```python
from build123d import *

# Parameters (mm, degrees)
RESSALTO_EXTRUS_O1_DEPTH   = 160
ESBO_O2_W                  = 7.6
ESBO_O2_H                  = 120
CORTE_EXTRUS_O1_DEPTH      = 30
CORTE_EXTRUS_O2_DEPTH      = 30
F_3DSKETCH3_R              = 2
CORTE_EXTRUS_O3_DEPTH      = 70
ESBO_O3_R                  = 6
ESBO_O3_W                  = 45.015344868
ESBO_O3_H                  = 129.478543367
ESBO_O3_W_2                = 37.192593828
CORTE_EXTRUS_O4_DEPTH      = 41
CORTE_EXTRUS_O4_DEPTH_BACK = 22


with BuildPart() as part:
    # Esboço1 → Ressalto-extrusão1 (new body)
    with BuildSketch(Plane.XY):
        with BuildLine():
            Line((-3.8, 21.821375341), (-3.8, -98.178624659))
            Line((-3.8, -98.178624659), (-5.7, -98.178624659))
            Line((-5.7, -98.178624659), (-5.360626179, -99.63308389))
            ThreePointArc((-5.360626179, -99.63308389), (-4.656141559, -100.745296045), (-3.41294376, -101.178624659))
            Line((-3.41294376, -101.178624659), (3.41294376, -101.178624659))
            ThreePointArc((3.41294376, -101.178624659), (4.656141559, -100.745296045), (5.360626179, -99.63308389))
            Line((5.360626179, -99.63308389), (5.7, -98.178624659))
            Line((5.7, -98.178624659), (3.8, -98.178624659))
            Line((3.8, -98.178624659), (3.8, 21.821375341))
            Line((3.8, 21.821375341), (5.7, 21.821375341))
            Line((5.7, 21.821375341), (4.013268169, 24.033911877))
            ThreePointArc((4.013268169, 24.033911877), (3.310139149, 24.613730366), (2.422747768, 24.821375341))
            Line((2.422747768, 24.821375341), (-2.297792791, 24.821375341))
            ThreePointArc((-2.297792791, 24.821375341), (-3.27177376, 24.568189891), (-3.999156919, 23.872736414))
            Line((-3.999156919, 23.872736414), (-5.266799243, 21.821375341))
            Line((-5.266799243, 21.821375341), (-3.8, 21.821375341))
        make_face()
    extrude(amount=RESSALTO_EXTRUS_O1_DEPTH)

    # Esboço2 → Corte-extrusão1 (cut)
    with BuildSketch(Plane.XY):
        with Locations((0, -38.178624659)):
            Rectangle(ESBO_O2_W, ESBO_O2_H)
    extrude(amount=CORTE_EXTRUS_O1_DEPTH, mode=Mode.SUBTRACT)

    # 3DSketch2 → Corte-extrusão2 (cut)
    with BuildSketch(Plane(origin=(-3.8, 21.821375341, 160), x_dir=(0.0632066956560733, -0.9980004577274705, 0), z_dir=(0, 0, -1))):
        Polygon((0, 0), (0.480370887, -7.584803479), (120.240425814, 0), (119.760054927, 7.584803479), align=None)
    extrude(amount=CORTE_EXTRUS_O2_DEPTH, mode=Mode.SUBTRACT)

    # 3DSketch3 → Corte-extrusão3 (cut)
    with BuildSketch(Plane(origin=(3.8, -38.178624659, 80), x_dir=(0, 0.7676852805184269, 0.6408270516101394), z_dir=(1, 0, 0))):
        with Locations(Location((0, 0, 0), (0, 0, 140.146481665))):
            Circle(F_3DSKETCH3_R)
        with Locations(Location((23.030558416, -19.224811548, 0), (0, 0, 140.146481665))):
            Circle(F_3DSKETCH3_R)
        with Locations(Location((-23.030558416, 19.224811548, 0), (0, 0, 140.146481665))):
            Circle(F_3DSKETCH3_R)
        with Locations(Location((-39.051234706, 0.032679535, 0), (0, 0, 140.146481665))):
            Circle(F_3DSKETCH3_R)
        with Locations(Location((-16.02067629, -19.192132013, 0), (0, 0, 140.146481665))):
            Circle(F_3DSKETCH3_R)
        with Locations(Location((7.009882125, -38.416943561, 0), (0, 0, 140.146481665))):
            Circle(F_3DSKETCH3_R)
        with Locations(Location((-6.982602808, 38.449623097, 0), (0, 0, 140.146481665))):
            Circle(F_3DSKETCH3_R)
        with Locations(Location((16.047955607, 19.224811548, 0), (0, 0, 140.146481665))):
            Circle(F_3DSKETCH3_R)
        with Locations(Location((39.078514023, 0, 0), (0, 0, 140.146481665))):
            Circle(F_3DSKETCH3_R)
    extrude(amount=-CORTE_EXTRUS_O3_DEPTH, mode=Mode.SUBTRACT)

    # Esboço3 → Corte-extrusão4 (cut, two sides)
    with BuildSketch(Plane(origin=(0, 0, 0), x_dir=(0, 0, -1), z_dir=(1, 0, 0))) as corte_extrus_o4_sk:
        with Locations(Location((-80, -38.178624659, 0), (0, 0, 270))):
            Circle(ESBO_O3_R)
        with Locations((-7.492327566, -39.917896343)):
            Rectangle(ESBO_O3_W, ESBO_O3_H)
        with Locations((-148.596296914, -39.917896343)):
            Rectangle(ESBO_O3_W_2, ESBO_O3_H)
    extrude(amount=CORTE_EXTRUS_O4_DEPTH, mode=Mode.SUBTRACT)
    extrude(corte_extrus_o4_sk.sketch, amount=-CORTE_EXTRUS_O4_DEPTH_BACK, mode=Mode.SUBTRACT)


solid = part.part
```
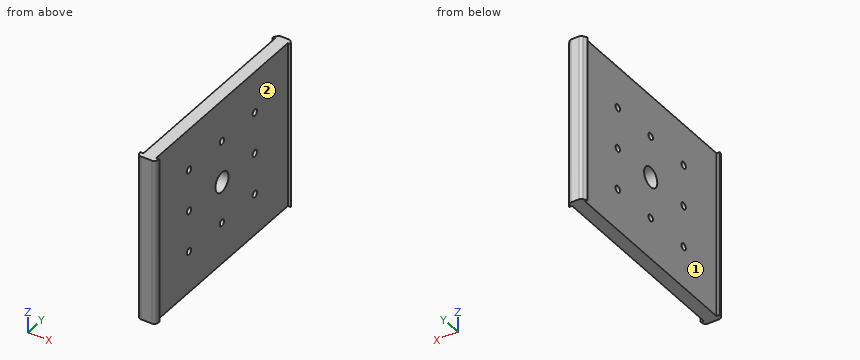
Read the model definition and answer for the solid it produces. Units are mm, in the model's axes. Face numbers are marked on the shaded views. A direction names the side the tool comes from. Give positions to 0.01 mm unless a question says otherwise; leave off trailing zeros. Write each loop counter-clockwise with the first axis right and the second up, starting at its lowest first coordinate (ties: lowest second). Pieces come first, ordered by that corner, then holes. Notation, with made-up numbers: (46.5, 45) - (70.5, 45) arc R18 ccw to (70.5, 50) - close; hole circle Ø3 at (74.25, 49.5). An arc over 180 degrees is marked (long way). Write item = value, one per line. Start each with the question number.
Item 1: A tool of negligible diameter and unlimited length cuts with its end or side. For the marked faces 1 and 2, from which of +Z, -Z, +X, -X, +Y, -Y can it reach the whole face along a straight path? Write none if from no direction.
Item 2: Find section D-D (y = -87). Give the vertices of the cut face in (x, z).
Item 3: Each of these flat-tipped pins is pushed along its axis until it touches: P1, Ø3.5, axis at y = -38.18, z = 55, coming from the +X side; P2, Ø1.6, axis at x = -4.5, z = 64, coming from the -Y side; P3, Ø1, axis at x = 4.5, z = 101, coming from the +Y side; P4, Ø5, axis at y = -68.18, z = 80, coming from the -X side. Where does it stop, or does it pass through?
Item 4: Find section A-A (z = 80). Give the vertices of the cut face in (x, y), then the cut area to 3 significant figures.
Item 5: Find section C-C (x = 1). State how many separate pieces and enclosed holes the cut face has, then the cut area to 3 significant figures.
Item 6: Find section B-B (z = 50.5). Give the vertices of the cut face in (x, y), then the cut area to 3 significant figures.
Item 7: Find the intervals of material crossed by probe 1 along Z at (x, y) = (-3.25, -8); probe 2 along Z at (x, y) = (0.75, -67); probe 3 along X at (y, z) = (-38.5, 123.5), in increasing order. Write a range as [from, to].
Response:
q1.face_1 = +Z, -Z, -X
q1.face_2 = +Z, -Z, +X
q2.outline = (-3.8, 30) - (3.8, 30) - (3.8, 130) - (-3.8, 130) - close
q3.P1 = through
q3.P2 = -101.16
q3.P3 = 24.05
q3.P4 = -3.8
q4.outline = (-5.7, -98.18) - (-5.36, -99.63) arc R2 ccw to (-3.41, -101.18) - (3.41, -101.18) arc R2 ccw to (5.36, -99.63) - (5.7, -98.18) - (3.8, -98.18) - (3.8, -70.18) - (-3.8, -70.18) - (-3.8, -98.18) - close; (-5.27, 21.82) - (-3.8, 21.82) - (-3.8, -6.18) - (3.8, -6.18) - (3.8, 21.82) - (5.7, 21.82) - (4.01, 24.03) arc R2 ccw to (2.42, 24.82) - (-2.3, 24.82) arc R2 ccw to (-4, 23.87) - close; (-3.8, -66.18) - (3.8, -66.18) - (3.8, -44.18) - (-3.8, -44.18) - close; (-3.8, -32.18) - (3.8, -32.18) - (3.8, -10.18) - (-3.8, -10.18) - close
q4.area = 817 mm²
q5.separate_pieces = 1
q5.enclosed_holes = 9
q5.area = 12,400 mm²
q6.outline = (-5.7, -98.18) - (-5.36, -99.63) arc R2 ccw to (-3.41, -101.18) - (3.41, -101.18) arc R2 ccw to (5.36, -99.63) - (5.7, -98.18) - (3.8, -98.18) - (3.8, 21.82) - (5.7, 21.82) - (4.01, 24.03) arc R2 ccw to (2.42, 24.82) - (-2.3, 24.82) arc R2 ccw to (-4, 23.87) - (-5.27, 21.82) - (-3.8, 21.82) - (-3.8, -98.18) - close
q6.area = 969 mm²
q7.probe_1 = [30, 53.01], [56.99, 78.01], [81.99, 103.05], [107.03, 130]
q7.probe_2 = [30, 53.38], [56.62, 78.38], [81.62, 103.43], [106.66, 130]
q7.probe_3 = [-3.8, 3.8]
